Geometry: final body of the model. Coordinates: model frame, mm. Face numbers are marked on the shaded views. A direction names the side the tool comes from. Give positions to 0.01 mm unless a question says otherwise; leave off trailing zeros. Write each loop counter-clockwise with the first axis right and the second up, starting at its lowest first coordinate (ties: lowest second). Pieces come first, ordered by that corner, then holes. Notation, with made-up numbers: (0.5, 18) -> (5.5, 18) arc R15 ccw to (5.5, 23) -> close; hole circle Ø4 at (-19.75, 67). An arc over 180 degrees is marked (long way). Answer as a JSON object with one key per item and string values. Group by question number.
(1) Section query C-C on z = 7.75. Output: boundary loops of the cut face in (x, y).
(2) Set-up query: the marked faces 1 and 2. Return all of +Z, -Z, +X, -X, +Y, -Y with unobstructed straight access to the full face (end or side cutting, diameter ignored); none if empty.
(3) Material intervals for probe 1 along Z at (x, y) = (27, -5); probe 2 along X at (y, z) = (4.25, 13.5); probe 3 along Z at (x, y) = (5, 0.5), sorted ascending.
(4) Section query B-B on y = -7. Output: boundary loops of the cut face in (x, z).
(5) Section query D-D on x = 14. Output: boundary loops of the cut face in (y, z).
(6) Contact query for flat-ended pins moving along their axis: pin 1 Ø8 at (y, z) = (-1, 17.5) entering from +X; pin 2 Ø1 at (x, z) = (13.5, 10.5) entering from +Y; pin 3 Ø3 at (x, y) = (15.5, 1) entering from +Z. Output: stop coordinate, or through.
from build123d import *

# Parameters (mm, degrees)
F1_DEPTH = 12.7
F2_R     = 12.7
F3_R     = 12.69999


# Not quite as in the source:
# - a fillet or chamfer is up to 0.001 mm smaller than in the source, because OpenCascade refuses the exact size


with BuildPart() as f1:
    # F0 (on Front) → F1 (new body, symmetric)
    with BuildSketch(Plane.XZ):
        Polygon((0, 25.4), (0, 0), (38.1, 0), (38.1, 6.35), (12.7, 6.35), (12.7, 25.4), align=None)
    extrude(amount=F1_DEPTH, both=True)

    # F2
    f2_edges = [f1.edges().sort_by_distance(p)[0] for p in [
        (6.35, -12.7, 25.4),
    ]]
    fillet(f2_edges, radius=F2_R)

    # F3 (radius 12.7 in the source; OpenCascade refuses exactly that, so slightly less here)
    f3_edges = [f1.edges().sort_by_distance(p)[0] for p in [
        (6.35, 12.7, 25.4),
    ]]
    fillet(f3_edges, radius=F3_R)


solid = f1.part
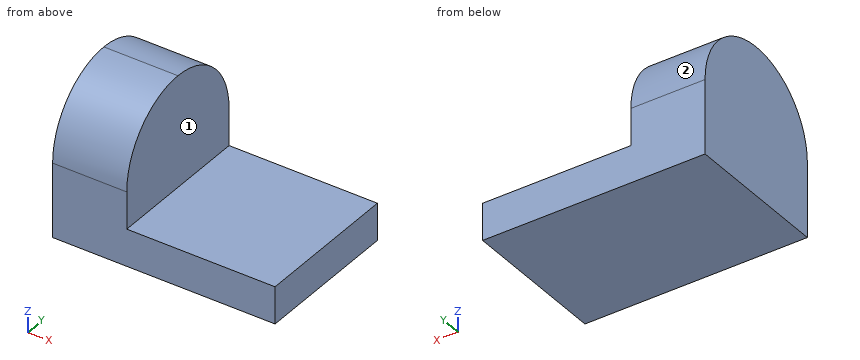
Answer list:
{
 "1": {"outline": "(0, -12.7) -> (12.7, -12.7) -> (12.7, 12.7) -> (0, 12.7) -> close"},
 "2": {"face 1": "+Z, +X, +Y, -Y", "face 2": "+Z, +X, -X, +Y"},
 "3": {"probe 1": "0 to 6.35", "probe 2": "0 to 12.7", "probe 3": "0 to 25.39"},
 "4": {"outline": "(0, 0) -> (38.1, 0) -> (38.1, 6.35) -> (12.7, 6.35) -> (12.7, 23.3) -> (0, 23.3) -> close"},
 "5": {"outline": "(-12.7, 0) -> (12.7, 0) -> (12.7, 6.35) -> (-12.7, 6.35) -> close"},
 "6": {"pin 1": "x = 12.7", "pin 2": "through", "pin 3": "z = 6.35"}
}
